from build123d import *

# Parameters (mm, degrees)
SWEEP_THIN1_PROFILE_R   = 55
SWEEP_THIN1_PROFILE_R_2 = 53
SKETCH69_W              = 300
SKETCH69_H              = 150
BOSS_EXTRUDE1_DEPTH     = 20


with BuildPart() as part:
    # Sweep-Thin1: sweep along a path in Sketch2
    with BuildLine(Plane(origin=(0, 0, 0), x_dir=(0, 0, -1), z_dir=(1, 0, 0))) as sweep_thin1_path:
        Line((0, 0), (0, 558.578643763))
        ThreePointArc((0, 558.578643763), (-7.612046749, 596.846986999), (-29.289321881, 629.289321881))
        Line((-29.289321881, 629.289321881), (-70.710678119, 670.710678119))
    # Sweep-Thin1 profile (on start of the path) → Sweep-Thin1 (sweep)
    with BuildSketch(Plane.ZX):
        Circle(SWEEP_THIN1_PROFILE_R)
        Circle(SWEEP_THIN1_PROFILE_R_2, mode=Mode.SUBTRACT)
    sweep(path=sweep_thin1_path.line)

    # Sketch69 → Boss-Extrude1 (add)
    with BuildSketch(Plane(origin=(0, 370.710678119, 370.710678119), x_dir=(1, 0, 0), z_dir=(0, 0.7071067811865489, 0.7071067811865461))):
        with Locations((0, 424.264068712)):
            Rectangle(SKETCH69_W, SKETCH69_H)
    extrude(amount=BOSS_EXTRUDE1_DEPTH)


solid = part.part
Could you check a few things on this model? Use its own coordinates, in mm. A direction names the side the tool comes from. Give positions to 0.01 mm unless a question says otherwise; leave off trailing zeros. Order: outer loops, then holes, each group sorted by start corner. A loop starts at its lowest first (then second) coordinate and runs counter-clockwise, first axis right, second up.
1. We'd pull the mould along Y, two halves only. Please class faces 1 (the flat face through (150, 677, 78)), 2 (the flat face through (-0.742, 671.235, 70.186)), 3 (the flat face through (-2.1, 624.65, 130.716)), 4 (the cylindrical face through (-33.47, 681.15, 19.43)): pulls with the +Y half, pulls with the -Y half, needs draft (parallel to the pull), parting line crosses it, or undercut.
2. Will these pins go through, and if not, where does the flat tip stop? P1, Ø10, axis at x = 55, y = 462.5, coming from the +Z side; P2, Ø1, axis at x = -21.5, z = 36, coming from the +Y side; P3, Ø6, axis at y = 91, z = 22, coming from the -X side.
3. Suppose I cut it at A-A (x = 0). List the corners of the cut face in (y, z) for me.
4. Suppose I cut it at B-B (y = 431.5). List the corners of the cut face in (x, z) for me, plus the area to 3 significant figures.
5. Suppose I cut it at C-C (x = -124.5). List the corners of the cut face in (y, z) for me, plus the area to 3 significant figures.
6. For faces 5 (the flat face through (-2.1, 685.595, 84.11)), 6 (the cylindrical face through (-53.692, 283.199, -11.923)), which set-ups out of +Z, -Z, +X, -X, +Y, -Y let a thin tool reach every point of the face, with its end or its side?
7. I need wall thicknesses on L1, parallel to X at y = 193, z = 0; L2, parallel to X at y = 75.5, z = 10; L3, parallel to Z at x = 8, y = 143. Which ranges of each line are inside material? Lowest first, please.
Solved:
1. face 1: needs draft
1. face 2: undercut
1. face 3: pulls with the -Y half
1. face 4: undercut
2. P1: stops at z = 22.91
2. P2: stops at y = 734.21
2. P3: stops at x = -51.61
3. outline: (0, -55) - (558.58, -55) arc R155 ccw to (668.18, -9.6) - (709.6, 31.82) - (723.74, 17.68) - (737.89, 31.82) - (631.82, 137.89) - (617.68, 123.74) - (631.82, 109.6) - (590.4, 68.18) arc R45 cw to (558.58, 55) - (0, 55) - (0, 53) - (558.58, 53) arc R47 ccw to (591.81, 66.77) - (633.23, 108.19) - (708.19, 33.23) - (666.77, -8.19) arc R153 cw to (558.58, -53) - (0, -53) - close
4. outline: circle Ø110 at (0, 0); hole circle Ø106 at (0, 0)
4. area: 679 mm2
5. outline: (617.68, 123.74) - (723.74, 17.68) - (737.89, 31.82) - (631.82, 137.89) - close
5. area: 3,000 mm2
6. face 5: +Z, +X, -X, +Y
6. face 6: -Y
7. L1: x = -55 to -53, 53 to 55
7. L2: x = -54.08 to -52.05, 52.05 to 54.08
7. L3: z = -54.42 to -52.39, 52.39 to 54.42
